Check sheet for the drawn part. Datum: minimum x, y, z corner. Units: mm. A direction names the side the tool comes from. Round coordinates to 2 decimals unless told otherwise and drop trailing zeros. Write each loop counter-clockwise with the first axis right and the second up, starting at its lowest first coordinate (ties: lowest second). Pieces come first, ordered by that corner, then holes. Notation, with made-up numbers: M 22.25,56 L 41.25,56 A13 cw 41.25,60 Z; hole C 53.25,65.25 d8. An arc over 180 degrees is marked long. Answer as CSV lines item,"result". Start each with the question number.
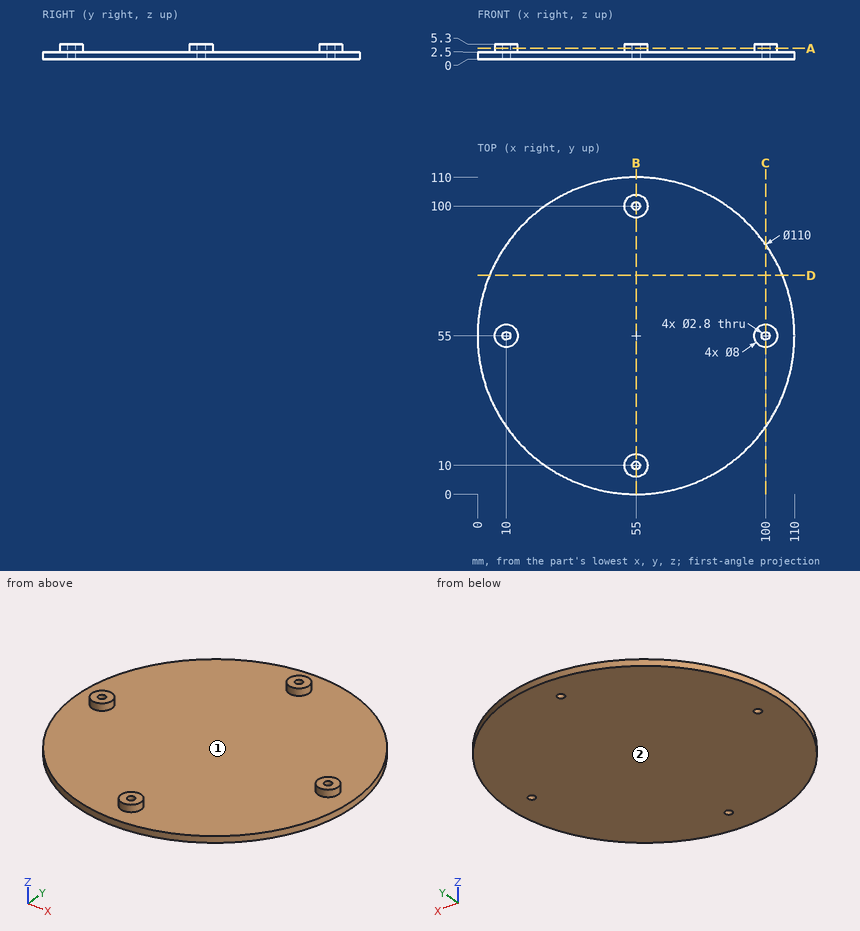
1) Go/stop test with flat-tipped pins: pin 1 (1.5 mm diameter, centred on x = 32, z = 2.5, fed in from -Y); pin 2 (1.5 mm diameter, centred on x = 45.5, y = 20.5, fed in from +Z); pin 3 (2 mm diameter, centred on y = 58.5, z = 4.5, fed in from -X). Record where each tip stops, or that it passes through.
2) Section check D-D, the plane y = 76. Record the cut outline in (x, z).
3) Scan lines: line 1 (X direction, y = 55, z = 3.25); line 2 (X direction, y = 10, z = 3.4). Record each from-to range of solid material in increasing order. Write a range as from..to.
4) Section check C-C, the plane x = 100. Record the cut outline in (y, z).
5) Section check B-B, the plane x = 55. Record the cut outline in (y, z).
6) Access from +Z, -Z, +X, -X, +Y, -Y to the whole of each face (thin tool, end or side, straight path). Record for the marked faces 1 and 2.
7) Section check A-A, the plane z = 3.8. Record the cut outline in (x, y), plus the area to 3 significant figures.
Results:
1,pin 1,"stops at y = 4.7"
1,pin 2,"stops at z = 2.5"
1,pin 3,"stops at x = 6.88"
2,outline,"M 4.17,0 L 105.83,0 L 105.83,2.5 L 4.17,2.5 Z"
3,line 1,"x = 6..8.6, 11.4..14, 96..98.6, 101.4..104"
3,line 2,"x = 51..53.6, 56.4..59"
4,outline,"M 23.38,0 L 53.6,0 L 53.6,5.3 L 51,5.3 L 51,2.5 L 23.38,2.5 Z; M 56.4,0 L 86.62,0 L 86.62,2.5 L 59,2.5 L 59,5.3 L 56.4,5.3 Z"
5,outline,"M 0,0 L 8.6,0 L 8.6,5.3 L 6,5.3 L 6,2.5 L 0,2.5 Z; M 11.4,0 L 98.6,0 L 98.6,5.3 L 96,5.3 L 96,2.5 L 14,2.5 L 14,5.3 L 11.4,5.3 Z; M 101.4,0 L 110,0 L 110,2.5 L 104,2.5 L 104,5.3 L 101.4,5.3 Z"
6,face 1,"+Z"
6,face 2,"-Z, +X, -X, +Y, -Y"
7,outline,"C 10,55 d8; C 55,10 d8; C 55,100 d8; C 100,55 d8; hole C 10,55 d2.8; hole C 55,10 d2.8; hole C 55,100 d2.8; hole C 100,55 d2.8"
7,area,"176 mm^2"
